CAD build for the part. Positions are in the model's coordinates, mm. A direction names the side the tool comes from. Give positions to 0.01 mm unless a question says otherwise; leave off trailing zeros. Write each loop counter-clockwise with the first axis right and the second up, starting at its lowest first coordinate (ties: lowest second). Pieces come first, ordered by that corner, then holes. Notation, with made-up numbers: M -16,-28 L 38,-28 A23 ccw 38,-10 Z; hole C -13,9.5 d3. An arc over 180 degrees is marked long. One line per question, with ' | ' between items. Start each with the question number.
1. Flat gauge pins, fed straight in: pin 1 (5 mm diameter, centred on x = 21, z = 3, fed in from -Y); pin 2 (4 mm diameter, centred on x = 23.5, y = -4, fed in from +Z); pin 3 (6 mm diameter, centred on x = 19.5, z = 6.5, fed in from +Y). Where does each tip first touch, or does it go through?
2. Which spindle directions (+Z, -Z, +X, -X, +Y, -Y) get a long thin tool onto all of the face, cutting with end or side? Do faces 1 (the face through (-3.743, 7.396, 4.19)), 2 (the face through (-0.4, -6, -5)). Say none if no direction does.
3. Wall check: L1, parallel to Z at x = 19, y = 1; L2, parallel to X at y = 1.25, z = 5.5; L3, parallel to X at y = -4.5, z = 6.5. Give the ranges that are in metal, low to high.
4. Cut at A-A, the plane x = 26. Write the cut outline in (y, z).
Autodesk Inventor part; units mm, degrees
ref_plane "Work Plane1" through (1.525, 0, 0) normal (0, 0, 1) x (1, 0, 0)
ref_plane "YZ Plane" through (0, 0, 0) normal (1, 0, 0) x (0, 1, 0)
ref_plane "XZ Plane" through (0, 0, 0) normal (0, 1, 0) x (-1, 0, 0)
sketch "Sketch1" plane through (0, 0, 0) normal (0, 0, 1) x (1, 0, 0)
  line L0 (0, 7.65) -> (0, 5)
  line L1 (6, 5) -> (32, 5)
  line L2 (32, 5) -> (32, 0)
  line L3 (32, 0) -> (-0.4001, 0)
  line L4 (-6.8801, 0) -> (38.48, 0)
  line L5 (-0.4001, 0) -> (-0.4001, 7.65)
  line L6 (-0.4001, 7.65) -> (0, 7.65)
  line L7 (6, 5) -> (5.0797, 5)
  line L8 (5.0797, 5) -> (0, 5)
  line L9 (0, -1.53) -> (0, 9.18)
  dimension "d0" = 32
  dimension "d1" = 26
  dimension "d2" = 10
  dimension "d9" = 0.4001
  dimension "d10" = 15.3
  dimension "d13" = 0.9203
  dimension "d14" = 10
revolve "Body" add sketch "Sketch1" angle 360 about axis through (32, 0, 0) along (-1, 0, 0)
sketch "Sketch2" plane through (-0.4001, 0, 0) normal (-1, 0, 0) x (0, 0, 1)
  line L0 (0, 9.815) -> (8.5, 4.9075)
  line L1 (8.5, 4.9075) -> (8.5, -4.9075)
  line L2 (8.5, -4.9075) -> (0, -9.815)
  line L3 (0, -9.815) -> (-8.5, -4.9075)
  line L4 (-8.5, -4.9075) -> (-8.5, 4.9075)
  line L5 (-8.5, 4.9075) -> (0, 9.815)
  point P0 (0, 0)
  point P1 (0, 0)
  dimension "d11" = 17
extrude "Head" add sketch "Sketch2" along normal blind 6.78
sketch "Sketch4" plane through (0, 0, 0) normal (0, 0, 1) x (1, 0, 0)
  line L0 (-7.1801, 8.5) -> (-7.1801, 9.815)
  line L1 (-7.1801, 9.815) -> (-6.4209, 9.815)
  line L2 (-6.4209, 9.815) -> (-7.1801, 8.5)
  line L3 (-8.5361, 0) -> (0.9559, 0)
  line L4 (-0.4001, 9.815) -> (-7.1801, 9.815)
  line L5 (-7.1801, 4.9075) -> (-7.1801, 9.815)
  dimension "d5" = 30
  dimension "d19" = 17
revolve "Chamfer1" cut sketch "Sketch4" angle 360 about axis through (-10, 0, 0) along (1, 0, 0)
thread "Thread"
chamfer "Chamfer2" distance 0.9202 distance2 0.9203 1 edges at (32, -5, 0) measured on face at (32, -0.2009, 0.1054)
ref_plane "Work Plane1" through (1.525, 0, 0) normal (0, 0, 1) x (1, 0, 0)
equation "\"d11\" = SW"
equation "\"d3\" = KOH - SD"
equation "\"d15\" = GEL"
equation "\"d6\" = -0.5 * SPD + 0.5 * GD"
equation "\"d0\" = NLG"
equation "\"d1\" = GEL"
equation "\"d2\" = GD"
equation "\"d10\" = SD2"
equation "\"d14\" = BDM"
equation "\"d5\" = ANG1"
equation "\"d19\" = SW0"
equation "\"NLG\" = 32"
equation "\"GD\" = NND"
equation "\"BDM\" = NND"
equation "\"KOH\" = 7.18"
equation "\"GEL\" = 26"
equation "\"SW\" = 17"
equation "\"SW0\" = 17"
equation "\"SPD\" = NND - 1.2269 * PTC"
equation "\"SD2\" = 0.9 * SW"
equation "\"SD\" = 0.4"
equation "\"ANG1\" = 30deg"
equation "\"GAL\" = 0.61345 * PTC"
equation "\"GUL\" = 0.61345 * PTC"
equation "\"RR\" = 0.6"
equation "\"GD1\" = THREADDIA - 1.2269 * PTC"
equation "\"SDH\" = 16.43"
equation "\"TOA\" = 30deg"
equation "\"PTC\" = 1.5"
equation "\"E0\" = 1.155 * SW"
properties part number "BS 3692 - M10 x 32" material "Steel, Mild"
Here are the results:
1) pin 1: y = -4.97 | pin 2: z = 4.58 | pin 3: y = 3.57
2) face 1: +Z, +X, -X, +Y | face 2: +X
3) L1: -4.9 to 4.9 | L2: -7.18 to 0 | L3: -7.18 to -0.4
4) outline: C 0,0 d10
